Check sheet for the modelled part. Datum: model origin and axes. Units: mm. A direction names the side the tool comes from. Give positions to 0.01 mm unless a question says otherwise; leave off trailing zeros. Loops run counter-clockwise (first coordinate to the right, second up) from the corner with the lowest first, then second, coordinate; pieces in that order, holes last. Notation, with made-up numbers: (14.5, 57) -> (49.5, 57) arc R17 ccw to (49.5, 71) -> close; hole circle Ø2 at (46.25, 4.25). An arc over 180 degrees is marked (long way). Answer as CSV lines item,"result". Start each with the question number.
(1) Gauge pin test, flat ends, axial feed: pin 1 Ø10.5 at (x, y) = (35, 53.5) entering from +Z; pin 2 Ø8 at (x, y) = (114.3, 50.8) entering from +Z. Record the tip position at first contact, or that the pin passes through.
(2) Material ranges on line 1 (Y direction, x = 82, z = 5.25) (3 decimals); line 2 (X direction, y = 93, z = 10); line 3 (X direction, y = 7.5, z = 1), recorded low to high. Write a range as from..to.
(3) Section check D-D on z = 9.25. State how many separate pieces and enclosed holes the cut face has, plus the area to 3 significant figures.
(4) Release check for a two-part mould opening along X. For faces 4 (the face through (109.34, 51.02, 3.78)), 5 (the face through (77, 101.6, 6)), 6 (the face through (1.91, 99.79, 5.89)) record: pulls with the +X half, pulls with the -X half, needs draft (parallel to the pull), parting line crosses it, or undercut.
(5) Section check C-C on x = 38.1. Enter the section's corners in (y, z).
(6) Section check B-B on x = 84. Enter the section's corners in (y, z) (3 decimals), plus the area to 3 significant figures.
(7) Section check A-A on y = 19.05. Enter the section's corners in (x, z) (3 decimals), plus the area to 3 significant figures.
(8) Access from +Z, -Z, +X, -X, +Y, -Y to the whole of each face (thin tool, end or side, straight path). Record for faces 1 (the face through (101.25, 41.53, 8)), 2 (the face through (60.326, 19.12, 6.439)), 3 (the face through (1.81, 1.91, 5.89)).
from build123d import *

# Parameters (mm, degrees)
EXTRUDE_1_DEPTH               = 12.7
SKETCH_2_R                    = 4.3053
CUT_EXTRUDE_1_DEPTH           = 184.601770144
CUT_EXTRUDE_2_DEPTH           = 184.601770144
SKETCH_4_R                    = 10.3124
CUT_EXTRUDE_3_DEPTH           = 7.9502
SKETCH_5_R                    = 6.7437
CUT_EXTRUDE_4_DEPTH           = 184.601770144
SKETCH_6_R                    = 9.525
CUT_EXTRUDE_5_DEPTH           = 5.244874679
CUT_EXTRUDE_5_DRAFT           = -41
SKETCH_7_R                    = 4.9657
CUT_EXTRUDE_6_DEPTH           = 184.601770144
SKETCH_8_R                    = 1.50495
CUT_EXTRUDE_7_DEPTH           = 9.525
SKETCH_9_R                    = 1.50495
CUT_EXTRUDE_8_DEPTH           = 0.901260886
CUT_EXTRUDE_8_DRAFT           = -59
CUT_EXTRUDE_8_PROFILE_2_DEPTH = 0.901260886
CUT_EXTRUDE_8_PROFILE_2_DRAFT = -59
CUT_EXTRUDE_8_PROFILE_3_DEPTH = 0.901260886
CUT_EXTRUDE_8_PROFILE_3_DRAFT = -59
CHAMFER_1_SIZE                = 0.762
CHAMFER_2_SIZE                = 0.762


with BuildPart() as part:
    # 草图1 → 凸台-拉伸1 (new body)
    with BuildSketch(Plane.XY):
        with BuildLine():
            Line((6.35, 0), (146.05, 0))
            ThreePointArc((146.05, 0), (150.540128061, 1.859871939), (152.4, 6.35))
            Line((152.4, 6.35), (152.4, 95.25))
            ThreePointArc((152.4, 95.25), (150.540128061, 99.740128061), (146.05, 101.6))
            Line((146.05, 101.6), (6.35, 101.6))
            ThreePointArc((6.35, 101.6), (1.859871939, 99.740128061), (0, 95.25))
            Line((0, 95.25), (0, 6.35))
            ThreePointArc((0, 6.35), (1.859871939, 1.859871939), (6.35, 0))
        make_face()
    extrude(amount=EXTRUDE_1_DEPTH)

    # 草图2 → 切除-拉伸1 (cut, through all)
    with BuildSketch(Plane.XY.offset(12.7)):
        with Locations((9.525, 9.525)):
            Circle(SKETCH_2_R)
        with Locations((142.875, 9.525)):
            Circle(SKETCH_2_R)
        with Locations((9.525, 92.075)):
            Circle(SKETCH_2_R)
        with Locations((142.875, 92.075)):
            Circle(SKETCH_2_R)
    extrude(amount=-CUT_EXTRUDE_1_DEPTH, mode=Mode.SUBTRACT)

    # 草图3 → 切除-拉伸2 (cut, through all)
    with BuildSketch(Plane.XY.offset(12.7)):
        with BuildLine():
            Line((63.5, 15.875), (88.9, 15.875))
            ThreePointArc((88.9, 15.875), (92.075, 19.05), (88.9, 22.225))
            Line((88.9, 22.225), (63.5, 22.225))
            ThreePointArc((63.5, 22.225), (60.325, 19.05), (63.5, 15.875))
        make_face()
    extrude(amount=-CUT_EXTRUDE_2_DEPTH, mode=Mode.SUBTRACT)

    # 草图4 → 切除-拉伸3 (cut)
    with BuildSketch(Plane.XY.offset(12.7)):
        with Locations((38.1, 50.8)):
            Circle(SKETCH_4_R)
    extrude(amount=-CUT_EXTRUDE_3_DEPTH, mode=Mode.SUBTRACT)

    # 草图5 → 切除-拉伸4 (cut, through all)
    with BuildSketch(Plane.XY.offset(12.7)):
        with Locations((38.1, 50.8)):
            Circle(SKETCH_5_R)
    extrude(amount=-CUT_EXTRUDE_4_DEPTH, mode=Mode.SUBTRACT)


with BuildPart() as cut_extrude_5_tool:
    # 草图6 → 切除-拉伸5 (with draft: the straight prism first)
    with BuildSketch(Plane.XY.offset(12.7)):
        with Locations((114.3, 50.8)):
            Circle(SKETCH_6_R)
    extrude(amount=-CUT_EXTRUDE_5_DEPTH)
    # 切除-拉伸5: the draft: its side faces are tilted about the plane it starts from
    cut_extrude_5_sides = [cut_extrude_5_tool.faces().sort_by_distance(p)[0] for p in [
        (104.775, 50.8, 10.07756266),
    ]]
    draft(cut_extrude_5_sides, Plane.XY.offset(12.7), CUT_EXTRUDE_5_DRAFT)


with BuildPart() as part_1:
    add(part.part)

    # 切除-拉伸5: cut by cut_extrude_5_tool
    add(cut_extrude_5_tool.part, mode=Mode.SUBTRACT)

    # 草图7 → 切除-拉伸6 (cut, through all)
    with BuildSketch(Plane.XY.offset(12.7)):
        with Locations((114.3, 50.8)):
            Circle(SKETCH_7_R)
    extrude(amount=-CUT_EXTRUDE_6_DEPTH, mode=Mode.SUBTRACT)

    # 草图8 → 切除-拉伸7 (cut)
    with BuildSketch(Plane.XY.offset(12.7)):
        with Locations((114.3, 66.675)):
            Circle(SKETCH_8_R)
        with Locations((100.551847, 42.8625)):
            Circle(SKETCH_8_R)
        with Locations((128.048153, 42.8625)):
            Circle(SKETCH_8_R)
    extrude(amount=-CUT_EXTRUDE_7_DEPTH, mode=Mode.SUBTRACT)


with BuildPart() as cut_extrude_8_tool:
    # 草图9 → 切除-拉伸8 (with draft: the straight prism first)
    with BuildSketch(Plane.XY.offset(3.175)):
        with Locations((114.3, 66.675)):
            Circle(SKETCH_9_R)
    extrude(amount=-CUT_EXTRUDE_8_DEPTH)
    # 切除-拉伸8: the draft: its side faces are tilted about the plane it starts from
    cut_extrude_8_sides = [cut_extrude_8_tool.faces().sort_by_distance(p)[0] for p in [
        (112.79505, 66.675, 2.724369557),
    ]]
    draft(cut_extrude_8_sides, Plane.XY.offset(3.175), CUT_EXTRUDE_8_DRAFT)


with BuildPart() as part_2:
    add(part_1.part)

    # 切除-拉伸8: cut by cut_extrude_8_tool
    add(cut_extrude_8_tool.part, mode=Mode.SUBTRACT)


with BuildPart() as cut_extrude_8_profile_2_tool:
    # 草图9 → 切除-拉伸8 profile 2 (with draft: the straight prism first)
    with BuildSketch(Plane.XY.offset(3.175)):
        with Locations((100.551847, 42.8625)):
            Circle(SKETCH_9_R)
    extrude(amount=-CUT_EXTRUDE_8_PROFILE_2_DEPTH)
    # 切除-拉伸8 profile 2: the draft: its side faces are tilted about the plane it starts from
    cut_extrude_8_profile_2_sides = [cut_extrude_8_profile_2_tool.faces().sort_by_distance(p)[0] for p in [
        (99.046897, 42.8625, 2.724369557),
    ]]
    draft(cut_extrude_8_profile_2_sides, Plane.XY.offset(3.175), CUT_EXTRUDE_8_PROFILE_2_DRAFT)


with BuildPart() as part_3:
    add(part_2.part)

    # 切除-拉伸8 profile 2: cut by cut_extrude_8_profile_2_tool
    add(cut_extrude_8_profile_2_tool.part, mode=Mode.SUBTRACT)


with BuildPart() as cut_extrude_8_profile_3_tool:
    # 草图9 → 切除-拉伸8 profile 3 (with draft: the straight prism first)
    with BuildSketch(Plane.XY.offset(3.175)):
        with Locations((128.048153, 42.8625)):
            Circle(SKETCH_9_R)
    extrude(amount=-CUT_EXTRUDE_8_PROFILE_3_DEPTH)
    # 切除-拉伸8 profile 3: the draft: its side faces are tilted about the plane it starts from
    cut_extrude_8_profile_3_sides = [cut_extrude_8_profile_3_tool.faces().sort_by_distance(p)[0] for p in [
        (126.543203, 42.8625, 2.724369557),
    ]]
    draft(cut_extrude_8_profile_3_sides, Plane.XY.offset(3.175), CUT_EXTRUDE_8_PROFILE_3_DRAFT)


with BuildPart() as part_4:
    add(part_3.part)

    # 切除-拉伸8 profile 3: cut by cut_extrude_8_profile_3_tool
    add(cut_extrude_8_profile_3_tool.part, mode=Mode.SUBTRACT)

    # 倒角1
    chamfer_1_edges = [part_4.edges().sort_by_distance(p)[0] for p in [
        (150.540128061, 1.859871939, 12.7),
        (152.4, 50.8, 12.7),
        (150.540128061, 99.740128061, 12.7),
        (76.2, 101.6, 12.7),
        (1.859871939, 99.740128061, 12.7),
        (0, 50.8, 12.7),
        (1.859871939, 1.859871939, 12.7),
        (76.2, 0, 12.7),
    ]]
    chamfer(chamfer_1_edges, length=CHAMFER_1_SIZE)

    # 倒角2
    chamfer_2_edges = [part_4.edges().sort_by_distance(p)[0] for p in [
        (138.5697, 9.525, 12.7),
        (5.2197, 92.075, 12.7),
        (138.5697, 92.075, 12.7),
        (5.2197, 9.525, 12.7),
    ]]
    chamfer(chamfer_2_edges, length=CHAMFER_2_SIZE)


solid = part_4.part
Working result:
1,pin 1,"stops at z = 4.75"
1,pin 2,"passes through"
2,line 1,"y = 0..15.875, 22.225..101.6"
2,line 2,"x = 0..5.32, 13.73..138.67, 147.08..152.4"
2,line 3,"x = 0..5.73, 13.32..139.08, 146.67..152.4"
3,separate pieces,"1"
3,enclosed holes,"10"
3,area,"14,500 mm^2"
4,face 4,"undercut"
4,face 5,"needs draft"
4,face 6,"pulls with the -X half"
5,outline,"(0, 0) -> (44.06, 0) -> (44.06, 4.75) -> (40.49, 4.75) -> (40.49, 12.7) -> (0.76, 12.7) -> (0, 11.94) -> close; (57.54, 0) -> (101.6, 0) -> (101.6, 11.94) -> (100.84, 12.7) -> (61.11, 12.7) -> (61.11, 4.75) -> (57.54, 4.75) -> close"
6,outline,"(0, 0) -> (15.875, 0) -> (15.875, 12.7) -> (0.762, 12.7) -> (0, 11.938) -> close; (22.225, 0) -> (101.6, 0) -> (101.6, 11.938) -> (100.838, 12.7) -> (22.225, 12.7) -> close"
6,area,"1,210 mm^2"
7,outline,"(0, 0) -> (60.325, 0) -> (60.325, 12.7) -> (0.762, 12.7) -> (0, 11.938) -> close; (92.075, 0) -> (152.4, 0) -> (152.4, 11.938) -> (151.638, 12.7) -> (92.075, 12.7) -> close"
7,area,"1,530 mm^2"
8,face 1,"+Z"
8,face 2,"+Z, -Z"
8,face 3,"+Z, -Z, -X, -Y"
